Geometry: final body of the model. Coordinates: model frame, mm. A direction names the side the tool comes from. Give positions to 0.01 mm unless a question says otherwise; leave off trailing zeros. Write each loop counter-clockwise with the first axis right and the second up, starting at its lowest first coordinate (ties: lowest second). Pieces come first, ordered by that corner, then holes. Notation, with made-up numbers: (-19.75, 9.25) -> (-12.75, 9.25) arc R23 ccw to (-12.75, 35.25) -> close; hole circle Ø4 at (78, 64.5). An arc over 180 degrees is marked (long way). Use CSV: the item, a comma, the result in double quotes. Start each with the question number.
1) Contact query for flat-ended pins moving along their axis: P1, Ø1.5, axis at y = 139.5, z = 1, coming from the -X side; P2, Ø4.5, axis at x = 125.29, y = 117.89, coming from the +Z side; P3, Ø3, axis at y = 77, z = 4, coming from the +X side; P4, Ø2, axis at x = 79, z = 5.5, coming from the -Y side. Output: stop coordinate, or through.
2) Section D-D (y = 77.5). Output: boundary loops of the cut face in (x, z), plus the area to 3 significant figures.
3) Section B-B (y = 145). Output: boundary loops of the cut face in (x, z), plus the area to 3 significant figures.
4) Set-up query: faces 5 (the face through (2.112, 60, 3)), 6 (the face through (-0.856, 143, 3)), 7 (the face through (-7.206, 113, 3)), 8 (the face through (140, 127.892, 3)), 9 (the face through (92.794, 41, 3)). Return all of +Z, -Z, +X, -X, +Y, -Y with unobstructed straight access to the full face (end or side cutting, diameter ignored); none if empty.
5) Material intervals for line 1 (Y direction, x = 13.5, z = 1.25); line 2 (Y direction, x = 126.5, z = 1.25); line 3 (Y direction, x = 69.5, z = 1.75), sorted ascending. Write a range as [from, to].
6) Section C-C (x = 23). Output: boundary loops of the cut face in (y, z), plus the area to 3 significant figures.
7) Section A-A (x = 115.5). Output: boundary loops of the cut face in (y, z), plus the area to 3 significant figures.
8) Draft query along Y for faces 1 (the face through (67, 44.242, 3)), 2 (the face through (68, 181.542, 3)), 3 (the face through (25, 50.892, 3)), 4 (the face through (92.794, 185, 3)). Return one class per face: pulls with the +Y half, pulls with the -Y half, needs draft (parallel to the pull), parting line crosses it, or undercut.
```python
from build123d import *

# Parameters (mm, degrees)
SKETCH2_R           = 49.5
SKETCH2_R_2         = 2.5
SKETCH2_R_3         = 1.095
SKETCH2_W           = 12
SKETCH2_H           = 19
SKETCH2_W_2         = 67
SKETCH2_H_2         = 7
BOSS_EXTRUDE1_DEPTH = 6.35


with BuildPart() as part:
    # Sketch2 → Boss-Extrude1 (new body)
    with BuildSketch(Plane.XY):
        Polygon((-7.205623902, 187.891798144), (-7.205623902, 157.891798144), (-0.855623902, 157.891798144), (-0.855623902, 127.891798144), (-7.205623902, 127.891798144), (-7.205623902, 97.891798144), (-0.855623902, 97.891798144), (-0.855623902, 67.891798144), (-7.205623902, 67.891798144), (-7.205623902, 37.891798144), (42.794376098, 37.891798144), (42.794376098, 44.241798144), (92.794376098, 44.241798144), (92.794376098, 37.891798144), (142.794376098, 37.891798144), (142.794376098, 67.891798144), (136.444376098, 67.891798144), (136.444376098, 97.891798144), (142.794376098, 97.891798144), (142.794376098, 127.891798144), (136.444376098, 127.891798144), (136.444376098, 157.891798144), (142.794376098, 157.891798144), (142.794376098, 187.891798144), (92.794376098, 187.891798144), (92.794376098, 181.541798144), (42.794376098, 181.541798144), (42.794376098, 187.891798144), align=None)
        with Locations((67.794376098, 117.891798144)):
            Circle(SKETCH2_R, mode=Mode.SUBTRACT)
        with Locations((38.181618431, 60.391798144)):
            Circle(SKETCH2_R_2, mode=Mode.SUBTRACT)
        with Locations((10.294376098, 117.891798144)):
            Circle(SKETCH2_R_2, mode=Mode.SUBTRACT)
        with Locations((67.794376098, 60.391798144)):
            Circle(SKETCH2_R_2, mode=Mode.SUBTRACT)
        with Locations((125.294376098, 117.891798144)):
            Circle(SKETCH2_R_2, mode=Mode.SUBTRACT)
        with Locations((67.794376098, 175.391798144)):
            Circle(SKETCH2_R_2, mode=Mode.SUBTRACT)
        with Locations((67.444376098, 52.660955737)):
            Circle(SKETCH2_R_3, mode=Mode.SUBTRACT)
        with Locations((138.444376098, 52.660955737)):
            Circle(SKETCH2_R_3, mode=Mode.SUBTRACT)
        with Locations((25.111805458, 60.391798144)):
            Rectangle(SKETCH2_W, SKETCH2_H, mode=Mode.SUBTRACT)
        with Locations((8.111805458, 60.391798144)):
            Rectangle(SKETCH2_W, SKETCH2_H, mode=Mode.SUBTRACT)
        with Locations((102.944376098, 52.660955737)):
            Rectangle(SKETCH2_W_2, SKETCH2_H_2, mode=Mode.SUBTRACT)
    extrude(amount=BOSS_EXTRUDE1_DEPTH)


solid = part.part
```
Answers follow:
1,P1,"stops at x = -0.86"
1,P2,"passes through"
1,P3,"stops at x = 136.44"
1,P4,"stops at y = 44.24"
2,outline,"(-0.86, 0) -> (39.18, 0) -> (39.18, 6.35) -> (-0.86, 6.35) -> close; (96.41, 0) -> (136.44, 0) -> (136.44, 6.35) -> (96.41, 6.35) -> close"
2,area,"508 mm^2"
3,outline,"(-0.86, 0) -> (26.38, 0) -> (26.38, 6.35) -> (-0.86, 6.35) -> close; (109.21, 0) -> (136.44, 0) -> (136.44, 6.35) -> (109.21, 6.35) -> close"
3,area,"346 mm^2"
4,face 5,"+Z, -Z"
4,face 6,"+Z, -Z, -X"
4,face 7,"+Z, -Z, -X, +Y, -Y"
4,face 8,"+Z, -Z, +X"
4,face 9,"+Z, -Z, -Y"
5,line 1,"y = [37.89, 50.89], [69.89, 187.89]"
5,line 2,"y = [37.89, 49.16], [56.16, 115.7], [120.08, 187.89]"
5,line 3,"y = [44.24, 49.16], [56.16, 58.56], [62.22, 68.42], [167.36, 173.56], [177.22, 181.54]"
6,outline,"(37.89, 0) -> (50.89, 0) -> (50.89, 6.35) -> (37.89, 6.35) -> close; (69.89, 0) -> (96.83, 0) -> (96.83, 6.35) -> (69.89, 6.35) -> close; (138.96, 0) -> (187.89, 0) -> (187.89, 6.35) -> (138.96, 6.35) -> close"
6,area,"564 mm^2"
7,outline,"(37.89, 0) -> (49.16, 0) -> (49.16, 6.35) -> (37.89, 6.35) -> close; (56.16, 0) -> (104.68, 0) -> (104.68, 6.35) -> (56.16, 6.35) -> close; (131.1, 0) -> (187.89, 0) -> (187.89, 6.35) -> (131.1, 6.35) -> close"
7,area,"740 mm^2"
8,face 1,"pulls with the -Y half"
8,face 2,"pulls with the +Y half"
8,face 3,"undercut"
8,face 4,"needs draft"
